Can you work these out from the model? Positions are in its coordinate system, mm. A direction names the side the tool comes from. Give positions to 0.01 mm unless a question says otherwise; leave off trailing zeros. Write each loop counter-clockwise with the first axis right and the second up, starting at its lowest first coordinate (ties: lowest second). Pieces come first, ordered by that corner, then holes. Notation, with made-up numbers: (57.5, 19) - (62.5, 19) arc R33 cw to (62.5, 50) - close; hole circle Ø5 at (65.5, 54.5). An arc over 180 degrees is marked (long way). Return JSON: item names as keys, results as strings. Group by question number.
from build123d import *

# Parameters (mm, degrees)
SKETCH1_W           = 80
SKETCH1_H           = 80
BOSS_EXTRUDE1_DEPTH = 4
BOSS_EXTRUDE2_DEPTH = 4


with BuildPart() as part:
    # Sketch1 → Boss-Extrude1 (new body)
    with BuildSketch(Plane(origin=(0, 0, 0), x_dir=(1, 0, 0), z_dir=(0, 1, 0))):
        Rectangle(SKETCH1_W, SKETCH1_H)
    extrude(amount=BOSS_EXTRUDE1_DEPTH)

    # Sketch2 → Boss-Extrude2 (add)
    with BuildSketch(Plane(origin=(0, 4, 0), x_dir=(1, 0, 0), z_dir=(0, 1, 0))):
        Polygon((-56.263455967, 37.878679656), (-40, 21.615223689), (-40, 40), (-21.615223689, 40), (-37.878679656, 56.263455967), align=None)
        Polygon((-37.878679656, -56.263455967), (-21.615223689, -40), (-40, -40), (-40, -21.615223689), (-56.263455967, -37.878679656), align=None)
        Polygon((40, 40), (40, 21.615223689), (56.263455967, 37.878679656), (37.878679656, 56.263455967), (21.615223689, 40), align=None)
        Polygon((21.615223689, -40), (37.878679656, -56.263455967), (56.263455967, -37.878679656), (40, -21.615223689), (40, -40), align=None)
    extrude(amount=-BOSS_EXTRUDE2_DEPTH)


solid = part.part
1) Imagine slicing it at C-C, the plane y = 2.95. Write out the boundary of the cut face in (x, z).
2) We'd pull the mould along X, two halves only. Please class faces 6 (the face through (-1, 4, -1)), 7 (the face through (29.633, 2.028, 48.018)), 8 (the face through (47.2, 2.03, -46.94)): pulls with the +X half, pulls with the -X half, needs draft (parallel to the pull), parting line crosses it, or undercut.
3) Imagine slicing it at D-D, the plane z = 6. Write out the boundary of the cut face in (x, y).
4) I need wall thicknesses on line 1 along Z through (x, y) = (-1.5, 3); line 2 along X through (y, z) = (0.35, -44.5). Which ranges of each line are inside material? Lowest first, please.
5) On a 3-axis mill with a long thin cutter (end or side, diameter ignored), from which of +Z, -Z, +X, -X, +Y, -Y can I reach the whole of each face in a straight line? I mean faces 1 (the face through (-40, 2, 0)), 2 (the face through (-1, 0, -1)), 3 (the face through (0, 2, -40)), 4 (the face through (40, 2, 0)), 5 (the face through (0, 2, 40)). Say none if no direction works.
6) Will these pins go through, and if not, where does the flat tip stop? pin 1 Ø1.5 at (y, z) = (1.5, -11.5) entering from -X; pin 2 Ø1.2 at (x, y) = (3.5, 2) entering from +Z; pin 3 Ø1.2 at (y, z) = (2.5, 1.5) entering from +X.
7) Imagine slicing it at B-B, the plane x = 43.5. Write out the boundary of the cut face in (y, z).
8) Imagine slicing it at A-A, the plane z = 42. Write out the boundary of the cut face in (x, y), and give its area (3 significant figures).
Resolved:
{
 "1": {"outline": "(-56.26, -37.88) - (-37.88, -56.26) - (-21.62, -40) - (21.62, -40) - (37.88, -56.26) - (56.26, -37.88) - (40, -21.62) - (40, 21.62) - (56.26, 37.88) - (37.88, 56.26) - (21.62, 40) - (-21.62, 40) - (-37.88, 56.26) - (-56.26, 37.88) - (-40, 21.62) - (-40, -21.62) - close"},
 "2": {"face 6": "needs draft", "face 7": "undercut", "face 8": "pulls with the +X half"},
 "3": {"outline": "(-40, 0) - (40, 0) - (40, 4) - (-40, 4) - close"},
 "4": {"line 1": "-40 to 40", "line 2": "-49.64 to -26.12, 26.12 to 49.64"},
 "5": {"face 1": "-X, +Y, -Y", "face 2": "+Z, -Z, +X, -X, -Y", "face 3": "-Z, +Y, -Y", "face 4": "+X, +Y, -Y", "face 5": "+Z, +Y, -Y"},
 "6": {"pin 1": "x = -40", "pin 2": "z = 40", "pin 3": "x = 40"},
 "7": {"outline": "(0, -50.64) - (4, -50.64) - (4, -25.12) - (0, -25.12) - close; (0, 25.12) - (4, 25.12) - (4, 50.64) - (0, 50.64) - close"},
 "8": {"outline": "(-52.14, 0) - (-23.62, 0) - (-23.62, 4) - (-52.14, 4) - close; (23.62, 0) - (52.14, 0) - (52.14, 4) - (23.62, 4) - close", "area": "228 mm^2"}
}
